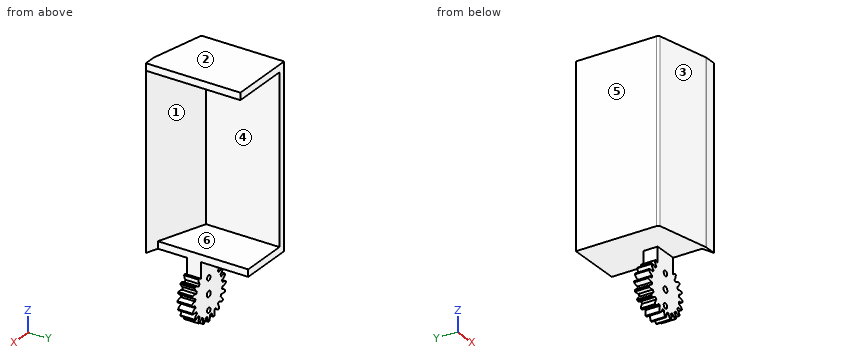
```python
from build123d import *

# Parameters (mm, degrees)
SKETCH_1_R          = 1.25
EXTRUDE_1_DEPTH     = 6
EXTRUDE_2_DEPTH     = 20
EXTRUDE_START       = -6
SKETCH_4_R          = 1.25
EXTRUDE_4_DEPTH     = 6
SKETCH_5_R          = 1.1
CUT_EXTRUDE_1_DEPTH = 97.337946833
EXTRUDE_5_DEPTH     = 76
CUT_EXTRUDE_2_DEPTH = 76


with BuildPart() as part:
    # 草图1 → 凸台-拉伸1 (new body)
    with BuildSketch(Plane(origin=(0, 0, 0), x_dir=(1, 0, 0), z_dir=(0, 1, 0))):
        with BuildLine():
            Line((5, 0), (5, -18))
            Line((5, -18), (-15, -18))
            Line((-15, -18), (-15, -88))
            Line((-15, -88), (10, -88))
            Line((10, -88), (10, -91))
            Line((10, -91), (-18, -91))
            Line((-18, -91), (-18, -15))
            Line((-18, -15), (-5, -15))
            Line((-5, -15), (-5, 0))
            ThreePointArc((-5, 0), (0, 5), (5, 0))
        make_face()
        with Locations(Location((0, 0, 0), (0, 0, 270))):
            Circle(SKETCH_1_R, mode=Mode.SUBTRACT)
    extrude(amount=-EXTRUDE_1_DEPTH)

    # 草图2 → 凸台-拉伸2 (add, symmetric)
    with BuildSketch(Plane(origin=(0, 0, 0), x_dir=(1, 0, 0), z_dir=(0, 1, 0))):
        Polygon((-15, -18), (5, -18), (5, -15), (-18, -15), (-18, -91), (10, -91), (10, -88), (-15, -88), align=None)
    extrude(amount=EXTRUDE_2_DEPTH, both=True)

    # 草图4 → 凸台-拉伸4 (add)
    with BuildSketch(Plane.XZ.offset(6).offset(EXTRUDE_START)):
        with BuildLine():
            ThreePointArc((0.860680542, 8.706562468), (0.72579344, 9.898750182), (0.24342364, 10.997306258))
            ThreePointArc((0.24342364, 10.997306258), (-0.01511058, 10.999989621), (-0.273636452, 10.996595977))
            ThreePointArc((-0.273636452, 10.996595977), (-0.752986286, 9.896718796), (-0.884597491, 8.704164996))
            ThreePointArc((-0.884597491, 8.704164996), (-1.380514283, 8.639397046), (-1.871919927, 8.546397884))
            ThreePointArc((-1.871919927, 8.546397884), (-2.368611449, 9.638553371), (-3.166844887, 10.53428182))
            ThreePointArc((-3.166844887, 10.53428182), (-3.413554747, 10.456942383), (-3.658378768, 10.373825947))
            ThreePointArc((-3.658378768, 10.373825947), (-3.77438681, 9.179653342), (-3.531037114, 8.00479718))
            ThreePointArc((-3.531037114, 8.00479718), (-3.982667613, 7.789952483), (-4.421283831, 7.549652329))
            ThreePointArc((-4.421283831, 7.549652329), (-5.231160146, 8.434867801), (-6.267120572, 9.040088481))
            ThreePointArc((-6.267120572, 9.040088481), (-6.477856391, 8.890296766), (-6.685013481, 8.735593555))
            ThreePointArc((-6.685013481, 8.735593555), (-6.426324056, 7.564019461), (-5.831834222, 6.521864044))
            ThreePointArc((-5.831834222, 6.521864044), (-6.194969688, 6.177973095), (-6.537861669, 5.813894202))
            ThreePointArc((-6.537861669, 5.813894202), (-7.58164644, 6.405518601), (-8.753926829, 6.660988295))
            ThreePointArc((-8.753926829, 6.660988295), (-8.908060318, 6.453406959), (-9.057272497, 6.242260401))
            ThreePointArc((-9.057272497, 6.242260401), (-8.449207929, 5.207966653), (-7.561770763, 4.400525414))
            ThreePointArc((-7.561770763, 4.400525414), (-7.800864967, 3.961250657), (-8.014468055, 3.509031603))
            ThreePointArc((-8.014468055, 3.509031603), (-9.189988356, 3.74915261), (-10.383837737, 3.629864165))
            ThreePointArc((-10.383837737, 3.629864165), (-10.466281235, 3.384812715), (-10.542942575, 3.137891306))
            ThreePointArc((-10.542942575, 3.137891306), (-9.64502446, 2.342121783), (-8.551508496, 1.848432697))
            ThreePointArc((-8.551508496, 1.848432697), (-8.643157232, 1.356773404), (-8.706562468, 0.860680542))
            ThreePointArc((-8.706562468, 0.860680542), (-9.898750182, 0.72579344), (-10.997306258, 0.24342364))
            ThreePointArc((-10.997306258, 0.24342364), (-10.999989621, -0.01511058), (-10.996595977, -0.273636452))
            ThreePointArc((-10.996595977, -0.273636452), (-9.896718796, -0.752986286), (-8.704164996, -0.884597491))
            ThreePointArc((-8.704164996, -0.884597491), (-8.639397046, -1.380514283), (-8.546397884, -1.871919927))
            ThreePointArc((-8.546397884, -1.871919927), (-9.638553371, -2.368611449), (-10.53428182, -3.166844887))
            ThreePointArc((-10.53428182, -3.166844887), (-10.456942383, -3.413554747), (-10.373825947, -3.658378768))
            ThreePointArc((-10.373825947, -3.658378768), (-9.179653342, -3.77438681), (-8.00479718, -3.531037114))
            ThreePointArc((-8.00479718, -3.531037114), (-7.789952483, -3.982667613), (-7.549652329, -4.421283831))
            ThreePointArc((-7.549652329, -4.421283831), (-8.434867801, -5.231160146), (-9.040088481, -6.267120572))
            ThreePointArc((-9.040088481, -6.267120572), (-8.890296766, -6.477856391), (-8.735593555, -6.685013481))
            ThreePointArc((-8.735593555, -6.685013481), (-7.564019461, -6.426324056), (-6.521864044, -5.831834222))
            ThreePointArc((-6.521864044, -5.831834222), (-6.177973095, -6.194969688), (-5.813894202, -6.537861669))
            ThreePointArc((-5.813894202, -6.537861669), (-6.405518601, -7.58164644), (-6.660988295, -8.753926829))
            ThreePointArc((-6.660988295, -8.753926829), (-6.453406959, -8.908060318), (-6.242260401, -9.057272497))
            ThreePointArc((-6.242260401, -9.057272497), (-5.207966653, -8.449207929), (-4.400525414, -7.561770763))
            ThreePointArc((-4.400525414, -7.561770763), (-3.961250657, -7.800864967), (-3.509031603, -8.014468055))
            ThreePointArc((-3.509031603, -8.014468055), (-3.74915261, -9.189988356), (-3.629864165, -10.383837737))
            ThreePointArc((-3.629864165, -10.383837737), (-3.384812715, -10.466281235), (-3.137891306, -10.542942575))
            ThreePointArc((-3.137891306, -10.542942575), (-2.342121783, -9.64502446), (-1.848432697, -8.551508496))
            ThreePointArc((-1.848432697, -8.551508496), (-1.356773404, -8.643157232), (-0.860680542, -8.706562468))
            ThreePointArc((-0.860680542, -8.706562468), (-0.72579344, -9.898750182), (-0.24342364, -10.997306258))
            ThreePointArc((-0.24342364, -10.997306258), (0.01511058, -10.999989621), (0.273636452, -10.996595977))
            ThreePointArc((0.273636452, -10.996595977), (0.752986286, -9.896718796), (0.884597491, -8.704164996))
            ThreePointArc((0.884597491, -8.704164996), (1.380514283, -8.639397046), (1.871919927, -8.546397884))
            ThreePointArc((1.871919927, -8.546397884), (2.368611449, -9.638553371), (3.166844887, -10.53428182))
            ThreePointArc((3.166844887, -10.53428182), (3.413554747, -10.456942383), (3.658378768, -10.373825947))
            ThreePointArc((3.658378768, -10.373825947), (3.77438681, -9.179653342), (3.531037114, -8.00479718))
            ThreePointArc((3.531037114, -8.00479718), (3.982667613, -7.789952483), (4.421283831, -7.549652329))
            ThreePointArc((4.421283831, -7.549652329), (5.231160146, -8.434867801), (6.267120572, -9.040088481))
            ThreePointArc((6.267120572, -9.040088481), (6.477856391, -8.890296766), (6.685013481, -8.735593555))
            ThreePointArc((6.685013481, -8.735593555), (6.426324056, -7.564019461), (5.831834222, -6.521864044))
            ThreePointArc((5.831834222, -6.521864044), (6.194969688, -6.177973095), (6.537861669, -5.813894202))
            ThreePointArc((6.537861669, -5.813894202), (7.58164644, -6.405518601), (8.753926829, -6.660988295))
            ThreePointArc((8.753926829, -6.660988295), (8.908060318, -6.453406959), (9.057272497, -6.242260401))
            ThreePointArc((9.057272497, -6.242260401), (8.449207929, -5.207966653), (7.561770763, -4.400525414))
            ThreePointArc((7.561770763, -4.400525414), (7.800864967, -3.961250657), (8.014468055, -3.509031603))
            ThreePointArc((8.014468055, -3.509031603), (9.189988356, -3.74915261), (10.383837737, -3.629864165))
            ThreePointArc((10.383837737, -3.629864165), (10.466281235, -3.384812715), (10.542942575, -3.137891306))
            ThreePointArc((10.542942575, -3.137891306), (9.64502446, -2.342121783), (8.551508496, -1.848432697))
            ThreePointArc((8.551508496, -1.848432697), (8.643157232, -1.356773404), (8.706562468, -0.860680542))
            ThreePointArc((8.706562468, -0.860680542), (9.898750182, -0.72579344), (10.997306258, -0.24342364))
            ThreePointArc((10.997306258, -0.24342364), (10.999989621, 0.01511058), (10.996595977, 0.273636452))
            ThreePointArc((10.996595977, 0.273636452), (9.896718796, 0.752986286), (8.704164996, 0.884597491))
            ThreePointArc((8.704164996, 0.884597491), (8.639397046, 1.380514283), (8.546397884, 1.871919927))
            ThreePointArc((8.546397884, 1.871919927), (9.638553371, 2.368611449), (10.53428182, 3.166844887))
            ThreePointArc((10.53428182, 3.166844887), (10.456942383, 3.413554747), (10.373825947, 3.658378768))
            ThreePointArc((10.373825947, 3.658378768), (9.179653342, 3.77438681), (8.00479718, 3.531037114))
            ThreePointArc((8.00479718, 3.531037114), (7.789952483, 3.982667613), (7.549652329, 4.421283831))
            ThreePointArc((7.549652329, 4.421283831), (8.434867801, 5.231160146), (9.040088481, 6.267120572))
            ThreePointArc((9.040088481, 6.267120572), (8.890296766, 6.477856391), (8.735593555, 6.685013481))
            ThreePointArc((8.735593555, 6.685013481), (7.564019461, 6.426324056), (6.521864044, 5.831834222))
            ThreePointArc((6.521864044, 5.831834222), (6.177973095, 6.194969688), (5.813894202, 6.537861669))
            ThreePointArc((5.813894202, 6.537861669), (6.405518601, 7.58164644), (6.660988295, 8.753926829))
            ThreePointArc((6.660988295, 8.753926829), (6.453406959, 8.908060318), (6.242260401, 9.057272497))
            ThreePointArc((6.242260401, 9.057272497), (5.207966653, 8.449207929), (4.400525414, 7.561770763))
            ThreePointArc((4.400525414, 7.561770763), (3.961250657, 7.800864967), (3.509031603, 8.014468055))
            ThreePointArc((3.509031603, 8.014468055), (3.74915261, 9.189988356), (3.629864165, 10.383837737))
            ThreePointArc((3.629864165, 10.383837737), (3.384812715, 10.466281235), (3.137891306, 10.542942575))
            ThreePointArc((3.137891306, 10.542942575), (2.342121783, 9.64502446), (1.848432697, 8.551508496))
            ThreePointArc((1.848432697, 8.551508496), (1.356773404, 8.643157232), (0.860680542, 8.706562468))
        make_face()
        with Locations(Location((0, 0, 0), (0, 0, 90))):
            Circle(SKETCH_4_R, mode=Mode.SUBTRACT)
    extrude(amount=EXTRUDE_4_DEPTH)

    # 草图5 → 切除-拉伸1 (cut, through all)
    with BuildSketch(Plane.XZ.offset(6)):
        with Locations(Location((0, 6.5, 0), (0, 0, 270))):
            Circle(SKETCH_5_R)
        with Locations(Location((0, -6.5, 0), (0, 0, 270))):
            Circle(SKETCH_5_R)
    extrude(amount=-CUT_EXTRUDE_1_DEPTH, mode=Mode.SUBTRACT)

    # 草图6 → 凸台-拉伸5 (add)
    with BuildSketch(Plane.XY.offset(91)):
        Polygon((-18, -10), (10, -20), (-18, -20), align=None)
    extrude(amount=-EXTRUDE_5_DEPTH)

    # 草图8 → 切除-拉伸2 (cut)
    with BuildSketch(Plane.XY.offset(91)):
        with BuildLine():
            Line((-17.212429644, -15.171210947), (4.895011274, -19.977176364))
            ThreePointArc((4.895011274, -19.977176364), (5.000614807, -19.994277719), (5.107440918, -20))
            Line((5.107440918, -20), (5.107440918, -20.306754101))
            Line((5.107440918, -20.306754101), (-18, -20.306754101))
            Line((-18, -20.306754101), (-18, -19.977176364))
            Line((-18, -19.977176364), (-18, -14.194034583))
            ThreePointArc((-18, -14.194034583), (-17.778597985, -14.821557633), (-17.212429644, -15.171210947))
        make_face()
    extrude(amount=-CUT_EXTRUDE_2_DEPTH, mode=Mode.SUBTRACT)


solid = part.part
```
Part model, mm, in its own coordinate system. Face numbers are marked on the shaded views. A direction names the side the tool comes from. Round coordinates to 2 decimals unless told otherwise and drop trailing zeros. Loops run counter-clockwise (first coordinate to the right, second up) from the corner with the lowest first, then second, coordinate; pieces in that order, holes last.
1. Slice it at A-A (z = 31). Give the cut face in (x, y), and give its area (3 significant figures).
Solutions:
outline: (-18, -14.19) arc R1 ccw to (-17.21, -15.17) - (4.9, -19.98) arc R1 ccw to (5.11, -20) - (10, -20) - (-15, -11.07) - (-15, 20) - (-18, 20) - close
area: 174 mm2
2. Two-plate mould, pull along Z, no slides. Class the marked faces 1, 2, 3 and 4: pulls with the +Z half, pulls with the -Z half, needs draft (parallel to the pull), parting line crosses it, or undercut.
Solutions:
face 1: undercut
face 2: pulls with the +Z half
face 3: needs draft
face 4: undercut
3. 3-axis set-ups, long thin cutter, end or side, ignore diameter. For the marked faces 5 and 6: which of +Z, -Z, +X, -X, +Y, -Y reach the whole face in a straight line?
Solutions:
face 5: +Z, -Z, -X, +Y, -Y
face 6: +X, +Y
4. Slice it at B-B (y = 10.5). Give the cut face in (x, z), and give its area (3 significant figures).
Solutions:
outline: (-18, 15) - (5, 15) - (5, 18) - (-15, 18) - (-15, 88) - (10, 88) - (10, 91) - (-18, 91) - close
area: 363 mm2
5. Slice it at C-C (y = -1.5). Count the separate pieces of the cut face and the enclosed holes in it, and give its area (3 significant figures).
Solutions:
separate pieces: 1
enclosed holes: 3
area: 711 mm2
6. Flat gauge pins, fed straight in: pin 1 (14 mm diameter, centred on x = -9, y = 6, fed in from -Z); pin 2 (1 mm diameter, centred on x = -11, z = 41.5, fed in from +Y); pin 3 (10.5 mm diameter, centred on y = -1, z = 14.5, fed in from +X). Where does each tip first touch, or does it go through?
Solutions:
pin 1: stops at z = -9.06
pin 2: stops at y = -12.32
pin 3: stops at x = 5
7. Drill centre lines: line 1 along X through (y, z) = (-3.3, 0); line 2 along Z through (x, y) = (-7.5, 16); line 3 along X through (y, z) = (-1, 6) (1 decimal). Where is each one in solid material? Low to high.
Solutions:
line 1: x = -11 to -1.25, 1.25 to 11
line 2: z = 15 to 18, 88 to 91
line 3: x = -9 to -6.8, -6.4 to -1, 1 to 6.4, 6.8 to 8.9
